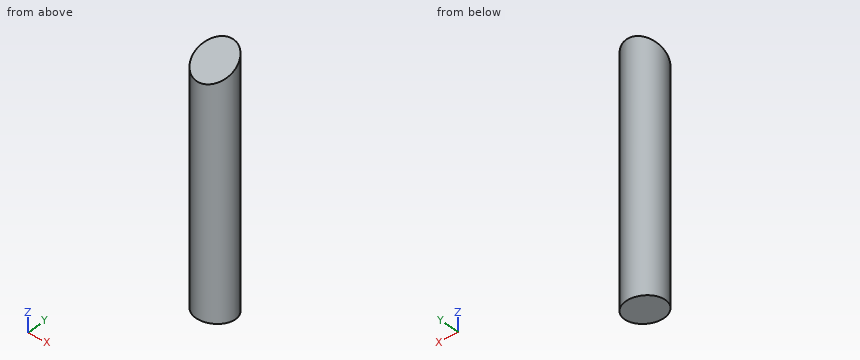
Autodesk Inventor part; units mm, degrees
ref_plane "Start Plane" through (0, 0, -1.0095) normal (0, 0, 1) x (1, 0, 0)
ref_plane "End Plane" through (0, 0, 123.7019) normal (0, 0, 1) x (1, 0, 0)
ref_plane "Work Plane4" through (0, 9.525, 123.7019) normal (0, -0.4462, 0.8949) x (1, 0, 0)
ref_plane "Start Plane" through (0, 0, -1.0095) normal (0, 0, 1) x (1, 0, 0)
ref_plane "End Plane" through (0, 0, 123.7019) normal (0, 0, 1) x (1, 0, 0)
sketch "Sketch" plane through (0, 0, 0) normal (0, 0, 1) x (1, 0, 0)
  circle A0 centre (0, 0) radius 9.525
  dimension "d0" = 19.05
extrude "Body" add sketch "Sketch" along normal up to surface (124.7114 mm away) from surface at -1.0095
sketch "Sketch2" plane through (0, 0, 0) normal (0, 0, 1) x (1, 0, 0)
  line L0 (0, 0) -> (10, 0)
ref_plane "Work Plane3" through (0, 0, 0) normal (0, -1, 0) x (1, 0, 0)
ref_plane "Work Plane4" through (0, 9.525, 123.7019) normal (0, -0.4462, 0.8949) x (1, 0, 0)
split "Split1" plane through (0, 9.525, 123.7019) removes the side toward (0, -0.4462, 0.8949)
ref_plane "Work Plane5" through (0, 9.525, -1.0095) normal (0, -0.1054, -0.9944) x (1, 0, 0)
split "Split2" plane through (0, 9.525, -1.0095) removes the side toward (0, -0.1054, -0.9944)
sketch "Sketch3" plane through (0, 0, 0) normal (0, -1, 0) x (1, 0, 0)
  line L0 (-2, -1.0095) -> (12, -1.0095)
  line L1 (-2, 123.7019) -> (12, 123.7019)
  dimension "d7" = 124.7114
equation "\"d0\" = Diam"
equation "\"d1\" = G_L"
equation "\"Diam\" = 19.05"
equation "\"G_L\" = d7"
equation "\"G_OFFSET_START\" = 1.00953"
equation "\"G_OFFSET_END\" = 4.74899"
equation "\"d4\" = -G_OFFSET_START"
equation "\"d5\" = G_OFFSET_END + B_L"
equation "\"B_L\" = 118.95289"
properties part number "ANSI/AISC Rolled Steel - 3/4-4.91, RB" material "Steel, Mild"
Geometry check sheet. Reference: the model listing, model coordinates, mm. Give positions to 0.01 mm unless a question says otherwise; leave off trailing zeros. Order: outer loops, then holes, each group sorted by start corner. A loop starts at its lowest first (then second) coordinate and runs counter-clockwise, first axis right, second up. Notation, with made-up numbers: (14.25, 82) - (36.25, 82) arc R25 ccw to (36.25, 111) - close; hole circle Ø6 at (-25.75, 13.5). An arc over 180 degrees is marked (long way). Write item = value, one per line. Start each with the question number.
1) Section check B-B (x = 0). Enter the section's corners in (y, z) (1 decimal).
2) Gauge pin test, flat ends, axial feed: pin 1 Ø8 at (x, z) = (-7, 46.5) entering from +Y; pin 2 Ø10 at (x, y) = (-7, -0.5) entering from -Z; pin 3 Ø10 at (x, y) = (-4, 5.5) entering from -Z. Record the tip position at first contact, or that the pin passes through.
3) Section check A-A (z = 74.5). Enter the section's corners in (x, y) (3 decimals), then the cut area to 3 significant figures.
4) Scan lines: L1, parallel to X at y = 0.25, z = 29; L2, parallel to Z at x = -2.25, y = -6; L3, parallel to Z at x = 3, y = 5.75. Record each from-to range of solid material in increasing order.
5) Section check C-C (y = 3). Enter the section's corners in (x, z), then the cut area to 3 significant figures.
Geometry check:
q1.outline = (-9.5, 1) - (9.5, -1) - (9.5, 123.7) - (-9.5, 114.2) - close
q2.pin_1 = 9.04
q2.pin_2 = -0.48
q2.pin_3 = -1
q3.outline = circle Ø19.05 at (0, 0)
q3.area = 285 mm2
q4.L1 = -9.52 to 9.52
q4.L2 = 0.64 to 115.96
q4.L3 = -0.61 to 121.82
q5.outline = (-9.04, -0.32) - (9.04, -0.32) - (9.04, 120.45) - (-9.04, 120.45) - close
q5.area = 2,180 mm2
